from build123d import *

# Parameters (mm, degrees)
PAD096_DEPTH       = 3
FILLET_R           = 0.5
CHAMFER061_SIZE    = 7
CHAMFER062_SIZE    = 0.4
CHAMFER062_FACE6_W = 15.5
CHAMFER062_FACE6_H = 3
PAD097_DEPTH       = 6
CHAMFER063_SIZE    = 1
FILLET065_R        = 8


with BuildPart() as part:
    # Sketch181 (on Binder) → Pad096 (new body)
    with BuildSketch(Plane.XY.offset(211.44686)):
        Polygon((-28.37148, 75), (-25.17148, 75), (-25.17148, 71.2), (-26.37148, 71.2), (-26.37148, 69), (-25.17148, 69), (-25.17148, 66), (-22.07148, 66), (-22.07148, 69), (-20.87148, 69), (-20.87148, 71.2), (-22.07148, 71.2), (-22.07148, 75), (-18.52148, 75), (-18.52148, 78.5), (-8.72148, 78.5), (-8.72148, 75), (-5.17148, 75), (-5.17148, 71.2), (-6.37148, 71.2), (-6.37148, 69), (-5.17148, 69), (-5.17148, 66), (-2.07148, 66), (-2.07148, 69), (-0.87148, 69), (-0.87148, 71.2), (-2.07148, 71.2), (-2.07148, 75), (1.12852, 75), (1.12852, 59), (-28.37148, 59), align=None)
    extrude(amount=PAD096_DEPTH)

    # Fillet
    fillet_edges = [part.edges().sort_by_distance(p)[0] for p in [
        (-18.52148, 78.5, 212.94686),
        (-8.72148, 78.5, 212.94686),
    ]]
    fillet(fillet_edges, radius=FILLET_R)

    # Chamfer061
    chamfer061_edges = [part.edges().sort_by_distance(p)[0] for p in [
        (1.12852, 59, 212.94686),
        (-28.37148, 59, 212.94686),
    ]]
    chamfer(chamfer061_edges, length=CHAMFER061_SIZE)

    # Chamfer062
    chamfer062_edges = [part.edges().sort_by_distance(p)[0] for p in [
        (-28.37148, 75, 212.94686),
        (1.12852, 75, 212.94686),
        (-2.07148, 75, 212.94686),
        (-5.17148, 75, 212.94686),
        (-22.07148, 75, 212.94686),
        (-25.17148, 75, 212.94686),
    ]]
    chamfer(chamfer062_edges, length=CHAMFER062_SIZE)

    # Chamfer062 Face6 → Pad097 (add)
    with BuildSketch(Plane(origin=(-13.62148, 59, 212.94686), x_dir=(-1, 0, 0), z_dir=(0, -1, 0))):
        Rectangle(CHAMFER062_FACE6_W, CHAMFER062_FACE6_H)
    extrude(amount=PAD097_DEPTH)

    # Chamfer063
    chamfer063_edges = [part.edges().sort_by_distance(p)[0] for p in [
        (-5.87148, 53, 212.94686),
        (-21.37148, 53, 212.94686),
    ]]
    chamfer(chamfer063_edges, length=CHAMFER063_SIZE)

    # Fillet065
    fillet065_edges = [part.edges().sort_by_distance(p)[0] for p in [
        (-21.37148, 59, 212.94686),
        (-28.37148, 66, 212.94686),
        (-5.87148, 59, 212.94686),
        (1.12852, 66, 212.94686),
    ]]
    fillet(fillet065_edges, radius=FILLET065_R)


solid = part.part
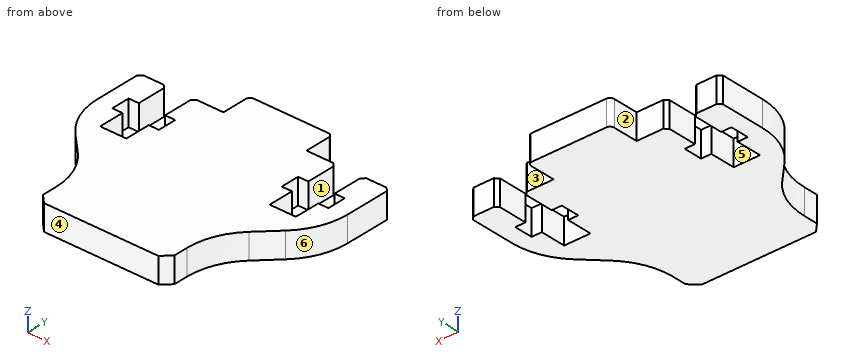
Source: CAD feature listing. Evaluate the final solid. Frame: model axes, mm. Face numbers are marked on the shaded views. A direction names the side the tool comes from. Coordinates: 2 decimals unless noted, no trailing zeros. Order: outer loops, then holes, each group sorted by start corner. A loop starts at its lowest first (then second) coordinate and runs counter-clockwise, first axis right, second up. Notation, with made-up numbers: M 9.25,18.5 L 56.25,18.5 A21 cw 56.25,36.5 Z; hole C 55,-11.5 d9. An arc over 180 degrees is marked long. Write each question's results on one line, items separated by ' | '. Start each with the question number.
1. Section B-B, the plane y = 55. Return the cut outline in (x, z).
2. Pin query (flat end, axial travel): pin 1 (1.5 mm diameter, centred on y = 55.5, z = 212.5, fed in from -X); pin 2 (0.6 mm diameter, centred on x = -21.5, z = 213, fed in from +Y); pin 3 (1.5 mm diameter, centred on x = -23, z = 213, fed in from +Y). Return the tip coordinate at first contact, or that it passes through.
3. Section A-A, the plane y = 68.5. Return the cut outline in (x, z), then the cut area to 3 significant figures.
4. Material intervals for L1, parallel to X at y = 73.75, z = 214.05; L2, parallel to X at y = 68.5, z = 214.15; L3, parallel to X at y = 55.25, z = 212.3, sorted ascending.
5. Section C-C, the plane y = 76.75. Return the cut outline in (x, z), then the cut area to 3 significant figures.
6. Draft query along X for the marked faces 4, 5 and 6. Return one class per face: +X half, -X half, draft (parallel to the pull), parting line (faces both ways), or undercut.
7. Reachability of the marked faces 1, 2 and 3 from +Z, -Z, +X, -X, +Y, -Y: full face, straight path, thin tool, end or side. Return the list, or none.
Solution:
1) outline: M -21.37,211.45 L -5.87,211.45 L -5.87,214.45 L -21.37,214.45 Z
2) pin 1: x = -21.39 | pin 2: y = 75 | pin 3: y = 66
3) outline: M -28.33,211.45 L -25.17,211.45 L -25.17,214.45 L -28.33,214.45 Z; M -22.07,211.45 L -5.17,211.45 L -5.17,214.45 L -22.07,214.45 Z; M -2.07,211.45 L 1.09,211.45 L 1.09,214.45 L -2.07,214.45 Z | area: 69.7 mm²
4) L1: -28.37 to -25.17, -22.07 to -5.17, -2.07 to 1.13 | L2: -28.33 to -25.17, -22.07 to -5.17, -2.07 to 1.09 | L3: -21.37 to -5.87
5) outline: M -18.52,211.45 L -8.72,211.45 L -8.72,214.45 L -18.52,214.45 Z | area: 29.4 mm²
6) face 4: draft | face 5: undercut | face 6: +X half
7) face 1: +Z, -Z, +Y | face 2: +Z, -Z, -X, +Y | face 3: +Z, -Z, +X, +Y
